For this review, take the finished solid that the model builds, in its own axes (mm). A direction names the side the tool comes from. Give positions to 0.01 mm unless a question says otherwise; leave off trailing zeros. Write each loop counter-clockwise with the first axis right and the second up, starting at its lowest first coordinate (ties: lowest second). Pieces come first, ordered by that corner, then holes.
1) We need section C-C on z = -5.5. Give the number of separate pieces and of enclosed holes in the cut face, and give its area (3 significant figures).
2) We need section B-B on x = 26.5. Give the boundary of the cut face in (y, z), and give its area (3 significant figures).
3) For P1, Ø10, axis at y = 42, z = -5.5, coming from the -X side; P2, Ø5, axis at x = 25, z = -18.5, coming from the +Y side; P3, Ø1, axis at x = 1.5, z = -33.5, coming from the +Y side; P4, Ø7.5, axis at x = -2.5, y = 27.5, coming from the +Z side, all flat-tipped, find the tip position at first contact; note any pin that passes through.
4) We need section D-D on y = 39.5. Give the boundary of the cut face in (x, z).
5) Machinability: for faces 1 (the face through (-20, 15, -20)), 2 (the face through (-9.713, 26.958, -14.64)), which of the approach directions +Z, -Z, +X, -X, +Y, -Y give a long, thin tool a straight path to every point of the face, cutting with its end or side? Answer none if there is none.
6) We need section A-A on y = 51. Give the boundary of the cut face in (x, z).
7) Wall thickness on line 1 along Z through (x, y) = (26.5, 21.75); line 2 along X through (y, z) = (28.1, -14.4); line 3 along Z through (x, y) = (26.5, 27.85): over which ranges is each line inside the solid? List them lowest first.
8) Draft analysis for pull direction Y (two halves, no side actions). For faces 3 (the face through (28.2, 26.6, -3.8)), 4 (the face through (20, 15, -20)), 5 (the face through (-0.448, 24.452, -4.923)), state which applies: pulls with the +Y half, pulls with the -Y half, needs draft (parallel to the pull), parting line crosses it, or undercut.
from build123d import *

# Parameters (mm, degrees)
SKETCH1_W                                           = 65
SKETCH1_H                                           = 41
BOSS_EXTRUDE1_DEPTH                                 = 16
SKETCH15_W                                          = 41
SKETCH15_H                                          = 10
BOSS_EXTRUDE4_DEPTH                                 = 23
SKETCH4_R                                           = 10.6
CUT_EXTRUDE3_DEPTH                                  = 11
M3_TAPPED_HOLE1_D                                   = 2.5
M3_TAPPED_HOLE1_DEPTH                               = 8.5
M3_TAPPED_HOLE1_TIP                                 = 0.751075774
CUT_EXTRUDE4_START                                  = -1
CUT_EXTRUDE4_DEPTH                                  = 1
SKETCH34_W                                          = 12.7
SKETCH34_H                                          = 2.6
CUT_EXTRUDE9_DEPTH                                  = 58.20576894
CUT_EXTRUDE7_DEPTH                                  = 1
M2_TAPPED_HOLE1_D                                   = 1.6
M2_TAPPED_HOLE1_DEPTH                               = 6
M2_TAPPED_HOLE1_TIP                                 = 0.480688495
CBORE_FOR_M4_HEX_SOCKET_HEAD_CAP_SCREW1_D           = 4.3
CBORE_FOR_M4_HEX_SOCKET_HEAD_CAP_SCREW1_CBORE_D     = 8
CBORE_FOR_M4_HEX_SOCKET_HEAD_CAP_SCREW1_CBORE_DEPTH = 4.4
FILLET1_R                                           = 5
CHAMFER4_SIZE                                       = 1
F_3_5_START                                         = 44
F_3_5_3_5_DIAMETER_SLOT1_DEPTH                      = 10
SKETCH33_W                                          = 15
SKETCH33_H                                          = 41
CUT_EXTRUDE8_DEPTH                                  = 2
CHAMFER5_SIZE                                       = 0.5


with BuildPart() as part:
    # Sketch1 → Boss-Extrude1 (new body)
    with BuildSketch(Plane(origin=(0, 15, 0), x_dir=(1, 0, 0), z_dir=(0, 1, 0))):
        with Locations((0, 20)):
            Rectangle(SKETCH1_W, SKETCH1_H)
    extrude(amount=BOSS_EXTRUDE1_DEPTH)

    # Sketch15 → Boss-Extrude4 (add)
    with BuildSketch(Plane(origin=(0, 31, 0), x_dir=(1, 0, 0), z_dir=(0, 1, 0))):
        with Locations((0, 4.5)):
            Rectangle(SKETCH15_W, SKETCH15_H)
    extrude(amount=BOSS_EXTRUDE4_DEPTH)

    # Sketch4 → Cut-Extrude3 (cut)
    with BuildSketch(Plane.XY.offset(0.5)):
        with Locations((1.85, 34.8)):
            Circle(SKETCH4_R)
    extrude(amount=-CUT_EXTRUDE3_DEPTH, mode=Mode.SUBTRACT)

    # M3 Tapped Hole1
    with Locations(Plane.XY.offset(0.5)):
        with Locations((13.974355653, 41.8), (1.85, 20.8), (-10.274355653, 41.8)):
            Hole(M3_TAPPED_HOLE1_D / 2, depth=M3_TAPPED_HOLE1_DEPTH)
            with Locations((0, 0, -(M3_TAPPED_HOLE1_DEPTH + M3_TAPPED_HOLE1_TIP / 2))):  # 118° drill point
                Cone(0, M3_TAPPED_HOLE1_D / 2, M3_TAPPED_HOLE1_TIP, mode=Mode.SUBTRACT)

    # Sketch16 → Cut-Extrude4 (cut)
    with BuildSketch(Plane(origin=(0, 31, 0), x_dir=(1, 0, 0), z_dir=(0, 1, 0)).offset(CUT_EXTRUDE4_START)):
        Polygon((-10.95, 12.5), (10.95, 12.5), (10.95, 16.3), (6.35, 16.3), (6.35, 37.9), (-6.35, 37.9), (-6.35, 16.3), (-10.95, 16.3), align=None)
    extrude(amount=CUT_EXTRUDE4_DEPTH, mode=Mode.SUBTRACT)

    # Sketch34 → Cut-Extrude9 (cut, through all)
    with BuildSketch(Plane(origin=(0, 30, 0), x_dir=(1, 0, 0), z_dir=(0, 1, 0))):
        with Locations((0, 39.2)):
            Rectangle(SKETCH34_W, SKETCH34_H)
    extrude(amount=CUT_EXTRUDE9_DEPTH, mode=Mode.SUBTRACT)

    # Sketch28 → Cut-Extrude7 (cut)
    with BuildSketch(Plane(origin=(0, 30, 0), x_dir=(1, 0, 0), z_dir=(0, 1, 0))):
        with BuildLine():
            Line((10.95, 12.5), (12.45, 12.5))
            ThreePointArc((12.45, 12.5), (13.510660172, 12.939339828), (13.95, 14))
            Line((13.95, 14), (13.95, 14.8))
            ThreePointArc((13.95, 14.8), (13.510660172, 15.860660172), (12.45, 16.3))
            Line((12.45, 16.3), (10.95, 16.3))
            Line((10.95, 16.3), (10.95, 12.5))
        make_face()
    cut_extrude7 = extrude(amount=CUT_EXTRUDE7_DEPTH, mode=Mode.SUBTRACT)

    # Mirror1: Cut-Extrude7 across plane
    add(cut_extrude7.mirror(Plane(origin=(0, 0, 0), x_dir=(0, 0, 1), z_dir=(1, 0, 0))), mode=Mode.SUBTRACT)

    # M2 Tapped Hole1
    with Locations(Plane(origin=(0, 30, 0), x_dir=(1, 0, 0), z_dir=(0, 1, 0))):
        with Locations((-4.45, 35.9), (4.45, 35.9), (8.95, 14.4), (-8.95, 14.4)):
            Hole(M2_TAPPED_HOLE1_D / 2, depth=M2_TAPPED_HOLE1_DEPTH)
            with Locations((0, 0, -(M2_TAPPED_HOLE1_DEPTH + M2_TAPPED_HOLE1_TIP / 2))):  # 118° drill point
                Cone(0, M2_TAPPED_HOLE1_D / 2, M2_TAPPED_HOLE1_TIP, mode=Mode.SUBTRACT)

    # CBORE for M4 Hex Socket Head Cap Screw1 (through all)
    with Locations(Plane(origin=(0, 31, 0), x_dir=(1, 0, 0), z_dir=(0, 1, 0))):
        with Locations((26.5, 34.5), (-26.5, 34.5), (-26.5, 5.5), (26.5, 5.5)):
            CounterBoreHole(CBORE_FOR_M4_HEX_SOCKET_HEAD_CAP_SCREW1_D / 2, CBORE_FOR_M4_HEX_SOCKET_HEAD_CAP_SCREW1_CBORE_D / 2, CBORE_FOR_M4_HEX_SOCKET_HEAD_CAP_SCREW1_CBORE_DEPTH)

    # Fillet1
    # the kernel refuses this fillet: 5 mm, written as the material it adds along each edge
    with BuildSketch(Plane(origin=(20.5, 31, 0.5), x_dir=(1, 0, 0), z_dir=(0, 0, -1))) as fillet1_piece_1_section:
        with BuildLine():
            CenterArc((FILLET1_R, -FILLET1_R), FILLET1_R, 90, 90)
            Line((0, -FILLET1_R), (0, 0))
            Line((0, 0), (FILLET1_R, 0))
        make_face()
    fillet1_piece_1 = extrude(amount=10, mode=Mode.PRIVATE)
    fillet1_piece_1 = fillet1_piece_1 - Plane(origin=(26.5, 31, -5.5), x_dir=(1, 0, 0), z_dir=(0, 1, 0)) * Cylinder(4, 41, mode=Mode.PRIVATE)
    add(fillet1_piece_1)
    with BuildSketch(Plane(origin=(-20.5, 31, -9.5), x_dir=(-1, 0, 0), z_dir=(0, 0, 1))) as fillet1_piece_2_section:
        with BuildLine():
            CenterArc((FILLET1_R, -FILLET1_R), FILLET1_R, 90, 90)
            Line((0, -FILLET1_R), (0, 0))
            Line((0, 0), (FILLET1_R, 0))
        make_face()
    fillet1_piece_2 = extrude(amount=10, mode=Mode.PRIVATE)
    fillet1_piece_2 = fillet1_piece_2 - Plane(origin=(-26.5, 31, -5.5), x_dir=(1, 0, 0), z_dir=(0, 1, 0)) * Cylinder(4, 41, mode=Mode.PRIVATE)
    add(fillet1_piece_2)

    # Chamfer4
    chamfer4_edges = [part.edges().sort_by_distance(p)[0] for p in [
        (-20.5, 54, -4.5),
        (20.5, 54, -4.5),
        (32.5, 23, 0.5),
        (-32.5, 23, 0.5),
        (32.5, 23, -40.5),
        (-32.5, 23, -40.5),
    ]]
    chamfer(chamfer4_edges, length=CHAMFER4_SIZE)

    # Ø3.5 (3.5) Diameter Slot1: read off the stored shape, not the designer's step
    # Ø3.5 (3.5) Diameter Slot1 outline → Ø3.5 (3.5) Diameter Slot1 (cut)
    with BuildSketch(Plane(origin=(0, 0, 0), x_dir=(1, 0, 0), z_dir=(0, 1, 0)).offset(F_3_5_START)):
        with BuildLine():
            Line((0.6, 0.8035), (3.1, 0.8035))
            ThreePointArc((3.1, 0.8035), (4.85, 2.5535), (3.1, 4.3035))
            Line((3.1, 4.3035), (0.6, 4.3035))
            ThreePointArc((0.6, 4.3035), (-1.15, 2.5535), (0.6, 0.8035))
        make_face()
    extrude(amount=F_3_5_3_5_DIAMETER_SLOT1_DEPTH, mode=Mode.SUBTRACT)

    # Sketch33 → Cut-Extrude8 (cut)
    with BuildSketch(Plane.XZ.offset(-15)):
        with Locations((0, -20)):
            Rectangle(SKETCH33_W, SKETCH33_H)
    extrude(amount=-CUT_EXTRUDE8_DEPTH, mode=Mode.SUBTRACT)

    # Chamfer5
    chamfer5_edges = [part.edges().sort_by_distance(p)[0] for p in [
        (7.5, 15, -20),
        (-7.5, 15, -20),
    ]]
    chamfer(chamfer5_edges, length=CHAMFER5_SIZE)


solid = part.part
Results list:
1. separate pieces: 3
1. enclosed holes: 4
1. area: 1,420 mm2
2. outline: (15, -40.5) - (31, -40.5) - (31, -38.5) - (26.6, -38.5) - (26.6, -36.65) - (15, -36.65) - close; (15, -32.35) - (26.6, -32.35) - (26.6, -30.5) - (31, -30.5) - (31, -9.5) - (26.6, -9.5) - (26.6, -7.65) - (15, -7.65) - close; (15, -3.35) - (26.6, -3.35) - (26.6, -1.5) - (31, -1.5) - (31, 0.5) - (15, 0.5) - close
2. area: 486 mm2
3. P1: stops at x = -20.5
3. P2: stops at y = 31
3. P3: stops at y = 30
3. P4: stops at z = 0.5
4. outline: (-20.5, -9.5) - (-7.65, -9.5) - (-7.65, 0.5) - (-20.5, 0.5) - close; (11.35, -9.5) - (20.5, -9.5) - (20.5, 0.5) - (11.35, 0.5) - close
5. face 1: +Z, -Z, +X, -X, -Y
5. face 2: +Y
6. outline: (-20.5, -9.5) - (20.5, -9.5) - (20.5, 0.5) - (-20.5, 0.5) - close; hole (0.6, -4.3) - (3.1, -4.3) arc R1.75 ccw to (3.1, -0.8) - (0.6, -0.8) arc R1.75 ccw to start
7. line 1: z = -40.5 to -36.65, -32.35 to -7.65, -3.35 to 0.5
7. line 2: x = -32.5 to -9.75, -8.15 to 8.15, 9.75 to 32.5
7. line 3: z = -40.5 to -38.5, -30.5 to -9.5, -1.5 to 0.5
8. face 3: pulls with the +Y half
8. face 4: pulls with the -Y half
8. face 5: undercut
